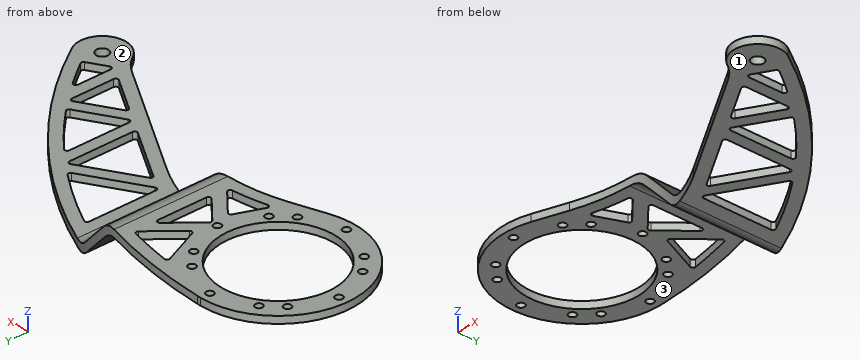
```python
from build123d import *

# Parameters (mm, degrees)
EXTRUDE_1_DEPTH          = 3
EXTRUDE_1_DEPTH_BACK     = 21
SKETCH_1_R               = 2.55
CUT_EXTRUDE_3_DEPTH      = 185.345637541
CUT_EXTRUDE_3_DEPTH_BACK = 185.345637541
SKETCH_2_R               = 1.55
CUT_EXTRUDE_1_DEPTH      = 185.711434636
SKETCH_4_R               = 1.55
CUT_EXTRUDE_2_DEPTH      = 185.711434636
FILLET_2_R               = 10
SKETCH_10_R              = 24
CUT_EXTRUDE_5_DEPTH      = 185.711434636
CUT_EXTRUDE_6_DEPTH      = 185.345637553
CUT_EXTRUDE_7_DEPTH      = 185.711434636


with BuildPart() as part:
    # 草图1 → 凸台-拉伸1 (new, two sides: drawn at the far end of the back side and taken through both)
    with BuildSketch(Plane.XY.offset(-EXTRUDE_1_DEPTH_BACK)):
        with BuildLine():
            Line((10.730362356, -31.206719208), (23.987000348, -26.648453139))
            ThreePointArc((23.987000348, -26.648453139), (58.3964084, -22.742948884), (91.232460283, -33.745404185))
            Line((91.232460283, -33.745404185), (142.367635598, -64.500382059))
            ThreePointArc((142.367635598, -64.500382059), (145.885654628, -67.188078585), (148.726187194, -70.583891486))
            ThreePointArc((148.726187194, -70.583891486), (162.505343691, -73.443257489), (165.49953058, -59.692767585))
            ThreePointArc((165.49953058, -59.692767585), (95.05641772, 7.182197604), (1.414573065, 32.983322541))
            ThreePointArc((1.414573065, 32.983322541), (0.707335687, 32.99583049), (0, 33))
            ThreePointArc((0, 33), (-32.548592395, -5.439589421), (10.730362356, -31.206719208))
        make_face()
        with Locations((157.059520527, -65.056183502)):
            Circle(SKETCH_1_R, mode=Mode.SUBTRACT)
    extrude(amount=EXTRUDE_1_DEPTH + EXTRUDE_1_DEPTH_BACK)

    # 草图6 → 切除-拉伸3 (cut, two sides: drawn at the far end of the back side and taken through both)
    with BuildSketch(Plane(origin=(0, 0, 0), x_dir=(1, 0, 0), z_dir=(0, 1, 0)).offset(-CUT_EXTRUDE_3_DEPTH_BACK)):
        with BuildLine():
            Line((-33, 0), (47.857864376, 0))
            ThreePointArc((47.857864376, 0), (51.6846987, 0.761204675), (54.928932188, 2.928932188))
            Line((54.928932188, 2.928932188), (73, 21))
            Line((73, 21), (-33, 21))
            Line((-33, 21), (-33, 0))
        make_face()
        with BuildLine():
            Line((53.242640687, -3), (71.313708499, 15.071067812))
            ThreePointArc((71.313708499, 15.071067812), (74.557941987, 17.238795325), (78.384776311, 18))
            Line((78.384776311, 18), (167.059520527, 18))
            Line((167.059520527, 18), (167.059520527, -3))
            Line((167.059520527, -3), (53.242640687, -3))
        make_face()
    extrude(amount=CUT_EXTRUDE_3_DEPTH + CUT_EXTRUDE_3_DEPTH_BACK, mode=Mode.SUBTRACT)

    # 草图2 → 切除-拉伸1 (cut, through all)
    with BuildSketch(Plane.XY.offset(3)):
        with Locations((-29, 0)):
            Circle(SKETCH_2_R)
        with Locations((0, -29)):
            Circle(SKETCH_2_R)
        with Locations((0, 29)):
            Circle(SKETCH_2_R)
        with Locations((29, 0)):
            Circle(SKETCH_2_R)
    extrude(amount=-CUT_EXTRUDE_1_DEPTH, mode=Mode.SUBTRACT)

    # 草图4 → 切除-拉伸2 (cut, through all)
    with BuildSketch(Plane.XY.offset(3)):
        with Locations((-22.388176755, 15.969331282)):
            Circle(SKETCH_4_R)
        with Locations((15.969331282, 22.388176755)):
            Circle(SKETCH_4_R)
        with Locations((-15.969331282, -22.388176755)):
            Circle(SKETCH_4_R)
        with Locations((22.388176755, -15.969331282)):
            Circle(SKETCH_4_R)
        with Locations((-15.969331282, 22.388176755)):
            Circle(SKETCH_4_R)
        with Locations((22.388176755, 15.969331282)):
            Circle(SKETCH_4_R)
        with Locations((15.969331282, -22.388176755)):
            Circle(SKETCH_4_R)
        with Locations((-22.388176755, -15.969331282)):
            Circle(SKETCH_4_R)
    extrude(amount=-CUT_EXTRUDE_2_DEPTH, mode=Mode.SUBTRACT)

    # 圆角2
    fillet_2_edges = [part.edges().sort_by_distance(p)[0] for p in [
        (73, -3.883124825, -21),
        (53.242640687, 1.256381871, 3),
    ]]
    fillet(fillet_2_edges, radius=FILLET_2_R)

    # 草图10 → 切除-拉伸5 (cut, through all)
    with BuildSketch(Plane.XY.offset(3)):
        Circle(SKETCH_10_R)
    extrude(amount=-CUT_EXTRUDE_5_DEPTH, mode=Mode.SUBTRACT)

    # 草图12 → 切除-拉伸6 (cut, through all)
    with BuildSketch(Plane.XY.offset(-18)):
        with BuildLine():
            Line((83.384776311, 6.091687583), (83.384776311, -22.39964463))
            ThreePointArc((83.384776311, -22.39964463), (83.884776311, -23.265670034), (84.884776311, -23.265670034))
            Line((84.884776311, -23.265670034), (109.047493079, -9.315319003))
            ThreePointArc((109.047493079, -9.315319003), (109.546460743, -8.494720534), (109.124030004, -7.632222505))
            ThreePointArc((109.124030004, -7.632222505), (97.246327471, 0.117641628), (84.83676315, 6.983712189))
            ThreePointArc((84.83676315, 6.983712189), (83.861319932, 6.943740058), (83.384776311, 6.091687583))
        make_face()
        with BuildLine():
            Line((113.281262253, -12.644453923), (90.464052196, -25.817976291))
            ThreePointArc((90.464052196, -25.817976291), (89.96414418, -26.697564816), (90.487726008, -27.563270347))
            ThreePointArc((90.487726008, -27.563270347), (92.159283091, -28.493281996), (93.809489051, -29.460672836))
            Line((93.809489051, -29.460672836), (113.2658565, -41.162601043))
            ThreePointArc((113.2658565, -41.162601043), (114.27349911, -41.176116075), (114.781262253, -40.305654774))
            Line((114.781262253, -40.305654774), (114.781262253, -13.510479327))
            ThreePointArc((114.781262253, -13.510479327), (114.281262253, -12.644453923), (113.281262253, -12.644453923))
        make_face()
        with BuildLine():
            Line((119.781262253, -17.831363982), (119.781262253, -43.349206201))
            ThreePointArc((119.781262253, -43.349206201), (120.281262253, -44.215231605), (121.281262253, -44.215231605))
            Line((121.281262253, -44.215231605), (138.118809565, -34.494069132))
            ThreePointArc((138.118809565, -34.494069132), (138.608354839, -33.7722663), (138.345198637, -32.940760006))
            ThreePointArc((138.345198637, -32.940760006), (130.119442072, -24.749716604), (121.420859845, -17.062654075))
            ThreePointArc((121.420859845, -17.062654075), (120.356761129, -16.925936572), (119.781262253, -17.831363982))
        make_face()
        with BuildLine():
            Line((126.148561535, -47.178597747), (141.15550656, -38.514333997))
            ThreePointArc((141.15550656, -38.514333997), (142.15550656, -38.514333997), (142.65550656, -39.3803594))
            Line((142.65550656, -39.3803594), (142.65550656, -57.070470024))
            ThreePointArc((142.65550656, -57.070470024), (142.147743417, -57.940931325), (141.140100807, -57.927416293))
            Line((141.140100807, -57.927416293), (126.133155781, -48.90156942))
            ThreePointArc((126.133155781, -48.90156942), (125.648601507, -48.035682123), (126.148561535, -47.178597747))
        make_face()
        with BuildLine():
            Line((147.65550656, -46.357104826), (147.65550656, -60.368443488))
            ThreePointArc((147.65550656, -60.368443488), (148.15550656, -61.234468891), (149.15550656, -61.234468891))
            Line((149.15550656, -61.234468891), (156.444782946, -57.026003208))
            ThreePointArc((156.444782946, -57.026003208), (156.920756292, -56.377867749), (156.765635798, -55.588838072))
            ThreePointArc((156.765635798, -55.588838072), (153.179787293, -50.604451681), (149.438785823, -45.73543482))
            ThreePointArc((149.438785823, -45.73543482), (148.326325199, -45.41283811), (147.65550656, -46.357104826))
        make_face()
    extrude(amount=-CUT_EXTRUDE_6_DEPTH, mode=Mode.SUBTRACT)

    # 草图13 → 切除-拉伸7 (cut, through all)
    with BuildSketch(Plane.XY.offset(3)):
        with BuildLine():
            Line((24.082747749, 24.562528501), (30.890663135, 9.020360956))
            ThreePointArc((30.890663135, 9.020360956), (31.658606615, 8.432604241), (32.56499258, 8.769738674))
            Line((32.56499258, 8.769738674), (43.039867443, 20.956056938))
            ThreePointArc((43.039867443, 20.956056938), (43.233300176, 21.914677314), (42.516477142, 22.579909593))
            ThreePointArc((42.516477142, 22.579909593), (33.868822783, 24.463648028), (25.144600346, 25.953057066))
            ThreePointArc((25.144600346, 25.953057066), (24.203957809, 25.570665357), (24.082747749, 24.562528501))
        make_face()
        with BuildLine():
            Line((44.100505063, -8.734608625), (44.100505063, 11.821995662))
            ThreePointArc((44.100505063, 11.821995662), (43.448103947, 12.759638993), (42.342155031, 12.473843212))
            Line((42.342155031, 12.473843212), (32.180437397, 0.651847549))
            ThreePointArc((32.180437397, 0.651847549), (31.941627156, -0.075308628), (32.28693988, -0.758350033))
            Line((32.28693988, -0.758350033), (42.448657514, -9.492958658))
            ThreePointArc((42.448657514, -9.492958658), (43.517729494, -9.64341211), (44.100505063, -8.734608625))
        make_face()
        with BuildLine():
            Line((32.585299227, -7.608069271), (42.290408687, -15.950195656))
            ThreePointArc((42.290408687, -15.950195656), (42.592011128, -17.01009687), (41.73578717, -17.703808015))
            ThreePointArc((41.73578717, -17.703808015), (34.703564931, -18.688791633), (27.778094538, -20.257294798))
            ThreePointArc((27.778094538, -20.257294798), (26.768536314, -19.955632396), (26.589551396, -18.917281582))
            Line((26.589551396, -18.917281582), (31.006342718, -7.991627393))
            ThreePointArc((31.006342718, -7.991627393), (31.69739783, -7.394679328), (32.585299227, -7.608069271))
        make_face()
    extrude(amount=-CUT_EXTRUDE_7_DEPTH, mode=Mode.SUBTRACT)


solid = part.part
```
Check sheet for the modelled part. Datum: model origin and axes. Units: mm. Face numbers are marked on the shaded views. A direction names the side the tool comes from. Coordinates: 2 decimals unless noted, no trailing zeros. Order: outer loops, then holes, each group sorted by start corner. A loop starts at its lowest first (then second) coordinate and runs counter-clockwise, first axis right, second up. Notation, with made-up numbers: M 24.5,82.5 L 49.5,82.5 A27 ccw 49.5,116.5 Z; hole C 2,59.5 d8. An arc over 180 degrees is marked long. One line per question, with ' | ' between items. Start each with the question number.
Item 1: Gauge pin test, flat ends, axial feed: P1, Ø6, axis at x = 137, z = -16, coming from the -Y side; P2, Ø1.5, axis at y = -53, z = -20, coming from the +X side; P3, Ø8, axis at x = 157.06, y = -65.06, coming from the +Z side; P4, Ø4, axis at x = -29, y = 0, coming from the +Z side. Record the tip position at first contact, or that the pin passes through.
Item 2: Material ranges on line 1 (Y direction, x = 29, z = 2.1); line 2 (X direction, y = -43, z = -19); line 3 (X direction, y = -42.5, z = -19), recorded low to high.
Item 3: Access from +Z, -Z, +X, -X, +Y, -Y to the whole of each face (thin tool, end or side, straight path). Record for the marked faces 1, 2 and 3.
Item 4: Sectioned sample at A-A on z = -7.25. Record the cut outline in (x, y), and give its area (3 significant figures).
Answer below:
1) P1: stops at y = -62.62 | P2: stops at x = 161.57 | P3: stops at z = -18 | P4: stops at z = 3
2) line 1: y = -25.11 to -19.94, -12.95 to -1.55, 1.55 to 13.34, 25.35 to 30.41 | line 2: x = 106.62 to 119.78, 123.39 to 133.39, 142.66 to 153.65 | line 3: x = 105.79 to 119.78, 124.25 to 134.25, 142.66 to 153.25
3) face 1: -Z, +X, -X, +Y, -Y | face 2: +Z, +X, +Y, -Y | face 3: -Z, -X, +Y, -Y
4) outline: M 59.25,-22.84 A80 cw 63.49,-23.45 L 63.49,21.56 A200 ccw 59.25,23.01 Z | area: 193 mm^2
